from build123d import *

# Parameters (mm, degrees)
F3_R     = 9.5
F3_R_2   = 7.5
F3_R_3   = 4.9
F4_DEPTH = 3
F5_DEPTH = 6
F6_DEPTH = 12.5


with BuildPart() as f4:
    # F3 (on Top) → F4 (new body)
    with BuildSketch(Plane.XY):
        Circle(F3_R)
        Circle(F3_R_2, mode=Mode.SUBTRACT)
        Circle(F3_R_2)
        Circle(F3_R_3, mode=Mode.SUBTRACT)
        Circle(F3_R_3)
        with BuildLine():
            ThreePointArc((-2.2847319318, -2.45), (-3.35, 0), (-2.2847319318, 2.45))
            Line((-2.2847319318, 2.45), (2.2847319318, 2.45))
            ThreePointArc((2.2847319318, 2.45), (3.35, 0), (2.2847319318, -2.45))
            Line((2.2847319318, -2.45), (-2.2847319318, -2.45))
        make_face(mode=Mode.SUBTRACT)
    extrude(amount=F4_DEPTH)

    # F3 (on Top) → F5 (join)
    with BuildSketch(Plane.XY):
        Circle(F3_R_2)
        Circle(F3_R_3, mode=Mode.SUBTRACT)
        Circle(F3_R_3)
        with BuildLine():
            ThreePointArc((-2.2847319318, -2.45), (-3.35, 0), (-2.2847319318, 2.45))
            Line((-2.2847319318, 2.45), (2.2847319318, 2.45))
            ThreePointArc((2.2847319318, 2.45), (3.35, 0), (2.2847319318, -2.45))
            Line((2.2847319318, -2.45), (-2.2847319318, -2.45))
        make_face(mode=Mode.SUBTRACT)
    extrude(amount=F5_DEPTH)

    # F3 (on Top) → F6 (join)
    with BuildSketch(Plane.XY):
        Circle(F3_R_3)
        with BuildLine():
            ThreePointArc((-2.2847319318, -2.45), (-3.35, 0), (-2.2847319318, 2.45))
            Line((-2.2847319318, 2.45), (2.2847319318, 2.45))
            ThreePointArc((2.2847319318, 2.45), (3.35, 0), (2.2847319318, -2.45))
            Line((2.2847319318, -2.45), (-2.2847319318, -2.45))
        make_face(mode=Mode.SUBTRACT)
    extrude(amount=F6_DEPTH)

    # F7 (on Front) → F8 (revolve)
    with BuildSketch(Plane.XZ):
        Polygon((5.15, 11.75), (4.9, 12.5), (4.9, 11), align=None)
    revolve(axis=Axis((0, 0, 8.7542282417), (0, 0, 1)))


solid = f4.part
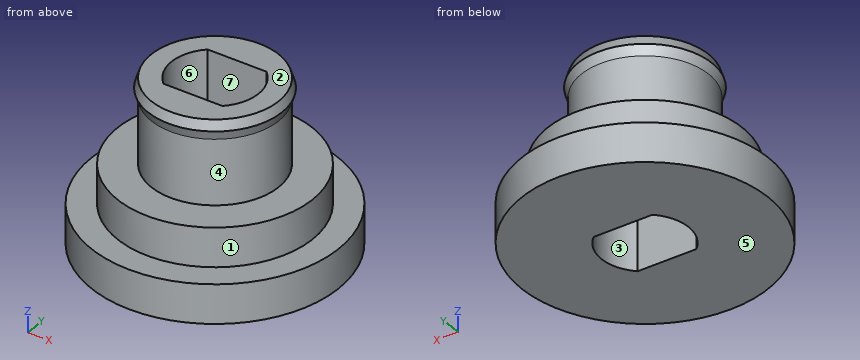
Input: part model. Units: mm. Frame: model coordinates. Face numbers are marked on the shaded views. A direction names the side the tool comes from. Coordinates: 2 decimals unless noted, no trailing zeros. Order: outer loops, then holes, each group sorted by start corner. A loop starts at its lowest first (then second) coordinate and runs counter-clockwise, first axis right, second up.
1. Contact query for flat-ended pins moving along their axis: P1, Ø5, axis at x = -7.5, z = 10, coming from the -Y side; P2, Ø2.5, axis at x = 1, z = 7.5, coming from the +Y side; P3, Ø1.4, axis at x = 0.5, z = 9, coming from the -Y side; P4, Ø2, axis at y = 3.5, z = 7.5, coming from the -X side. Output: stop coordinate, or through.
Checked values:
P1: passes through
P2: stops at y = 4.9
P3: stops at y = -4.9
P4: stops at x = -4.21
2. Access query for the marked faces 1, 2 and 3. Directions: +Z, -Z, +X, -X, +Y, -Y. A direction counts if a zero-diameter tool reaches every point of the face in a straight line with its end or side. Return the directions, or none.
Checked values:
face 1: +Z
face 2: +Z, +X, -X, +Y, -Y
face 3: +Z, -Z
3. Cut plane D-D, the plane y = 6.5. Return loops of the section in (x, z).
Checked values:
outline: (-6.93, 0) - (6.93, 0) - (6.93, 3) - (3.74, 3) - (3.74, 6) - (-3.74, 6) - (-3.74, 3) - (-6.93, 3) - close
4. Ray query, line 1 along Y through (x, z) = (-0.75, 2.5); line 2 along Y through (x, z) = (-1.5, 9.25); line 3 along Z through (x, y) = (7, -5.5). Return the intervals inside material, ascending.
Checked values:
line 1: y = -9.47 to -2.45, 2.45 to 9.47
line 2: y = -4.66 to -2.45, 2.45 to 4.66
line 3: z = 0 to 3
5. Cut plane C-C, the plane z = 3.5. Return loops of the section in (x, y).
Checked values:
outline: circle Ø15 at (0, 0); hole (-2.28, -2.45) - (2.28, -2.45) arc R3.35 ccw to (2.28, 2.45) - (-2.28, 2.45) arc R3.35 ccw to start
6. Cut plane A-A, the plane x = 0. Return loops of the section in (y, z).
Checked values:
outline: (-9.5, 0) - (-2.45, 0) - (-2.45, 12.5) - (-4.9, 12.5) - (-5.15, 11.75) - (-4.9, 11) - (-4.9, 6) - (-7.5, 6) - (-7.5, 3) - (-9.5, 3) - close; (2.45, 0) - (9.5, 0) - (9.5, 3) - (7.5, 3) - (7.5, 6) - (4.9, 6) - (4.9, 11) - (5.15, 11.75) - (4.9, 12.5) - (2.45, 12.5) - close
7. Cut plane B-B, the plane y = 0. Return loops of the section in (x, z).
Checked values:
outline: (-9.5, 0) - (-3.35, 0) - (-3.35, 12.5) - (-4.9, 12.5) - (-5.15, 11.75) - (-4.9, 11) - (-4.9, 6) - (-7.5, 6) - (-7.5, 3) - (-9.5, 3) - close; (3.35, 0) - (9.5, 0) - (9.5, 3) - (7.5, 3) - (7.5, 6) - (4.9, 6) - (4.9, 11) - (5.15, 11.75) - (4.9, 12.5) - (3.35, 12.5) - close
8. Draft query along X for the marked faces 4, 5, 6 and 7. Return one class per face: +X half, -X half, draft (parallel to the pull), parting line (faces both ways), or undercut.
Checked values:
face 4: parting line
face 5: draft
face 6: undercut
face 7: undercut
